Could you check a few things on this model? Use its own coordinates, in mm. Face numbers are marked on the shaded views. A direction names the side the tool comes from. Coordinates: 2 decimals unless noted, no trailing zeros. Order: outer loops, then holes, each group sorted by start corner. A loop starts at its lowest first (then second) coordinate and runs counter-clockwise, first axis right, second up. Notation, with made-up numbers: (43.25, -17) - (48.25, -17) arc R27 cw to (48.25, 16) - close; hole circle Ø7 at (-31.75, 3.25). An arc over 180 degrees is marked (long way). One line per item, written item: value.
Autodesk Inventor part; units mm, degrees
ref_plane "YZ Plane" through (0, 0, 0) normal (1, 0, 0) x (0, 1, 0)
ref_plane "XZ Plane" through (0, 0, 0) normal (0, 1, 0) x (-1, 0, 0)
ref_plane "XY Plane" through (0, 0, 0) normal (0, 0, 1) x (1, 0, 0)
sketch "Sketch1" plane through (0, 0, 0) normal (0, 0, 1) x (1, 0, 0)
  line L0 (-17.1448, -21) -> (23.7, -21)
  line L1 (23.7, -21) -> (23.7, -13)
  line L2 (23.7, -13) -> (12.3117, -13)
  line L3 (12.3117, -13) -> (12.3117, -14)
  line L4 (12.3117, -14) -> (3.1793, -16)
  line L5 (3.1793, -16) -> (-10.1347, -16)
  line L6 (-10.1347, -16) -> (-10.1347, -14.8234)
  arc A0 (-10.1347, -14.8234) -> (-14.1347, -10.8234) centre (-14.1347, -14.8234) ccw
  line L7 (-14.1347, -10.8234) -> (-17.1448, -10.8234)
  arc A1 (-17.1448, -10.8234) -> (-21.1448, -14.8234) centre (-17.1448, -14.8234) ccw
  line L8 (-21.1448, -14.8234) -> (-21.1448, -17)
  arc A2 (-21.1448, -17) -> (-17.1448, -21) centre (-17.1448, -17) ccw
  circle A3 centre (-15.5, -15.5) radius 1.5
  circle A4 centre (15.3552, -15.5) radius 1.5
  point P0 (0, 0)
extrude "Extrusion1" add sketch "Sketch1" along normal blind 3
sketch "Sketch2" plane through (0, 0, 3) normal (0, 0, 1) x (1, 0, 0)
  circle A0 centre (15.3552, -15.5) radius 1.5
  line L0 (-10, -16) -> (-10, -21)
  line L1 (23.7, -21) -> (-10, -21)
  line L2 (23.7, -13) -> (23.7, -21)
  line L3 (12.3117, -13) -> (23.7, -13)
  line L4 (12.3117, -14) -> (12.3117, -13)
  line L5 (3.1793, -16) -> (12.3117, -14)
  line L6 (-10, -16) -> (3.1793, -16)
  circle A1 centre (15.5, -15.5) radius 1.5
  point P0 (0, 0)
extrude "Extrusion2" add sketch "Sketch2" along normal blind 14
sketch "Sketch4" plane through (0, 0, 17) normal (0, 0, 1) x (1, 0, 0)
  line L0 (-10, -16) -> (-10, -21)
  line L1 (-10, -21) -> (23.7, -21)
  line L2 (23.7, -21) -> (23.7, -13)
  line L3 (23.7, -13) -> (12.3117, -13)
  line L4 (12.3117, -13) -> (12.3117, -14)
  line L5 (12.3117, -14) -> (3.1793, -16)
  line L6 (3.1793, -16) -> (-10, -16)
  arc A0 (15.4276, -14.0017) -> (15.4276, -16.9983) centre (15.3552, -15.5) ccw
  arc A1 (15.4276, -16.9983) -> (15.4276, -14.0017) centre (15.5, -15.5) ccw
  line L7 (-10, -21) -> (-10, -16)
  line L8 (-10, -16) -> (-10.1347, -16)
  line L9 (-10.1347, -16) -> (-10.1347, -14.8234)
  arc A2 (-10.1347, -14.8234) -> (-14.1347, -10.8234) centre (-14.1347, -14.8234) ccw
  line L10 (-14.1347, -10.8234) -> (-17.1448, -10.8234)
  arc A3 (-17.1448, -10.8234) -> (-21.1448, -14.8234) centre (-17.1448, -14.8234) ccw
  line L11 (-21.1448, -14.8234) -> (-21.1448, -17)
  arc A4 (-21.1448, -17) -> (-17.1448, -21) centre (-17.1448, -17) ccw
  line L12 (-17.1448, -21) -> (-10, -21)
  circle A5 centre (-15.5, -15.5) radius 1.5
  point P0 (0, 0)
extrude "Extrusion3" add sketch "Sketch4" along normal blind 3
sketch "Sketch5" plane through (-17.1448, -21, 0) normal (0, -1, 0) x (1, 0, 0)
  line L0 (7.1448, 3) -> (7.1448, 17)
  circle A0 centre (12.889, 3.3484) radius 2.5
  circle A1 centre (12.889, 9.9795) radius 2.5
  line L1 (8.5448, -0.0205) -> (17.5875, -0.0205)
  line L2 (17.5875, -0.0205) -> (17.5875, 14.0778)
  line L3 (17.5875, 14.0778) -> (8.5448, 14.0778)
  line L4 (8.5448, 14.0778) -> (8.5448, -0.0205)
  point P0 (17.1448, 0)
  point P1 (17.1448, -14)
  dimension "d6" = 5
  dimension "d8" = 5
  dimension "d9" = 4.0983
  dimension "d10" = 4.6985
  dimension "d11" = 3.3689
  dimension "d12" = 4.3442
  dimension "d13" = 6.6311
  dimension "d14" = 1.4
extrude "Extrusion4" add sketch "Sketch5" along normal blind 10
sketch "Sketch6" plane through (-4.2558, -21, 9.9795) normal (0, -1, 0) x (1, 0, 0)
  circle A0 centre (0, 0) radius 2.5
  circle A1 centre (0, 0) radius 1
  point P0 (4.2558, -9.9795)
  dimension "d17" = 2
extrude "Extrusion5" cut sketch "Sketch6" against normal blind 10 contours A1
sketch "Sketch7" plane through (-17.1448, -21, 0) normal (0, -1, 0) x (1, 0, 0)
  line L0 (17.5875, 0) -> (40.8448, 0)
  line L1 (40.8448, 0) -> (40.8448, 20)
  circle A0 centre (36.5448, 10) radius 4
  point P0 (17.1448, 0)
  dimension "d21" = 4.3
  dimension "d22" = 10
  dimension "d23" = 8
extrude "Extrusion6" cut sketch "Sketch7" against normal blind 1
sketch "Sketch8" plane through (19.4, -20, 10) normal (0, -1, 0) x (1, 0, 0)
  circle A0 centre (0, 0) radius 4
  circle A1 centre (0, 0) radius 2
  point P0 (-19.4, -10)
  dimension "d26" = 4
extrude "Extrusion7" cut sketch "Sketch8" against normal blind 11 contours A1
properties part number "exTop"
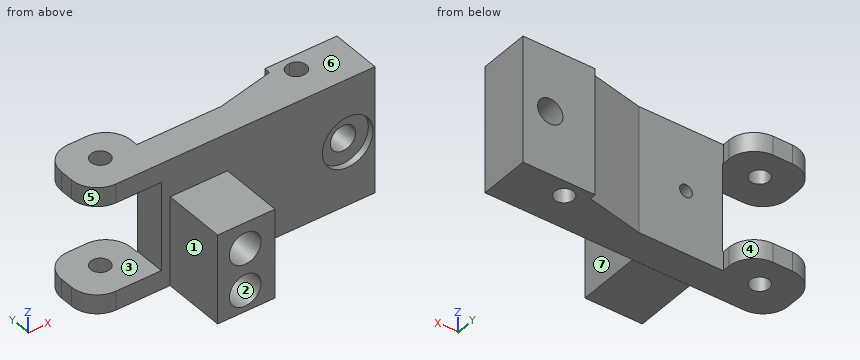
Item 1: For the marked faces 1, 2 and 3, which set-ups out of +Z, -Z, +X, -X, +Y, -Y let a thin tool reach every point of the face, with its end or its side?
Conclusion:
face 1: +Z, -Z, -X, -Y
face 2: -Y
face 3: -X, +Y, -Y
Item 2: I want a section at D-D on z = 17.75. Please give me the cut outline in (x, y).
Conclusion:
outline: (-21.14, -17) arc R4 ccw to (-17.14, -21) - (23.7, -21) - (23.7, -13) - (12.31, -13) - (12.31, -14) - (3.18, -16) - (-10.13, -16) - (-10.13, -14.82) arc R4 ccw to (-14.13, -10.82) - (-17.14, -10.82) arc R4 ccw to (-21.14, -14.82) - close; hole circle Ø3 at (-15.5, -15.5); hole (15.43, -17) arc R1.5 ccw (long way) to (15.43, -14) arc R1.5 ccw (long way) to start
Item 3: I want a section at C-C on x = -15.5. Please give me the cut outline in (y, z), then the cut area to 3 significant figures.
Conclusion:
outline: (-21, 0) - (-17, 0) - (-17, 3) - (-21, 3) - close; (-21, 17) - (-17, 17) - (-17, 20) - (-21, 20) - close; (-14, 0) - (-10.82, 0) - (-10.82, 3) - (-14, 3) - close; (-14, 17) - (-10.82, 17) - (-10.82, 20) - (-14, 20) - close
area: 43.1 mm²
Item 4: Thinking about a two-plate mould opening in X: for the marked faces 4, 5, 6 and 7, which applies, pulls with the +X half, pulls with the -X half, needs draft (parallel to the pull), parting line crosses it, or undercut?
Conclusion:
face 4: undercut
face 5: pulls with the -X half
face 6: needs draft
face 7: pulls with the +X half
Item 5: I want a section at B-B on y = -15.5. Give the number of separate pieces and of enclosed holes in the cut face, then the cut area to 3 significant figures.
Conclusion:
separate pieces: 6
enclosed holes: 1
area: 338 mm²
Item 6: If I drill on probe 1 along Z at (x, y) = (19.4, -20.7); probe 2 along X at (y, z) = (-18.75, 12.5); probe 3 along Y at (x, z) = (14.5, 9.25), over which ranges is the centre line in solid material (lowest first)?
Conclusion:
probe 1: 0 to 6, 14 to 20
probe 2: -10 to 23.7
probe 3: -21 to -16.73, -14.27 to -13
Item 7: I'm going to push flat-ended pins straight in: pin 1 Ø4 at (x, y) = (-15.5, -15.5) entering from -Z; pin 2 Ø8 at (x, z) = (-4.26, 3.35) entering from +Y; pin 3 Ø8 at (x, z) = (15.5, 16.5) entering from +Y; pin 4 Ø8 at (x, z) = (-4.26, 9.98) entering from -Y. Where does each tip first touch, or does it pass through?
Conclusion:
pin 1: z = 0
pin 2: y = -16
pin 3: y = -13
pin 4: y = -31
Item 8: I want a section at A-A on x = 19.4. Please give me the cut outline in (y, z).
Conclusion:
outline: (-21, 0) - (-13, 0) - (-13, 8) - (-20, 8) - (-20, 6) - (-21, 6) - close; (-21, 14) - (-20, 14) - (-20, 12) - (-13, 12) - (-13, 20) - (-21, 20) - close
